from build123d import *

# Parameters (mm, degrees)
BOSS_EXTRUDE1_DEPTH                            = 6.35
CSK_FOR_4_FLAT_HEAD_MACHINE_SCREW1_D           = 3.2639
CSK_FOR_4_FLAT_HEAD_MACHINE_SCREW1_CSINK_D     = 5.715
CSK_FOR_4_FLAT_HEAD_MACHINE_SCREW1_CSINK_ANGLE = 82
CSK_FOR_4_FLAT_HEAD_MACHINE_SCREW2_D           = 3.2639
CSK_FOR_4_FLAT_HEAD_MACHINE_SCREW2_CSINK_D     = 5.715
CSK_FOR_4_FLAT_HEAD_MACHINE_SCREW2_CSINK_ANGLE = 82
CHAMFER1_SIZE                                  = 10.558581723
CHAMFER1_SIZE_2                                = 6.096
CUT_EXTRUDE1_REACH                             = 697.184
SKETCH8_W                                      = 25.4
SKETCH8_H                                      = 49.00517421
CSK_FOR_4_FLAT_HEAD_MACHINE_SCREW3_D           = 3.2639
CSK_FOR_4_FLAT_HEAD_MACHINE_SCREW3_CSINK_D     = 5.715
CSK_FOR_4_FLAT_HEAD_MACHINE_SCREW3_CSINK_ANGLE = 82


with BuildPart() as part:
    # Sketch1 → Boss-Extrude1 (new body)
    with BuildSketch(Plane(origin=(0, 0, 0), x_dir=(0, 0, -1), z_dir=(1, 0, 0))):
        with BuildLine():
            Line((-123.515928009, -106.162611625), (-0.699091996, 106.562388375))
            ThreePointArc((-0.699091996, 106.562388375), (110.865451078, 218.126931449), (263.265451078, 258.962388375))
            Line((263.265451078, 258.962388375), (646.089089029, 258.962388375))
            Line((646.089089029, 258.962388375), (646.089089029, -106.162611625))
            Line((646.089089029, -106.162611625), (-123.515928009, -106.162611625))
        make_face()
    extrude(amount=BOSS_EXTRUDE1_DEPTH)

    # CSK for #4 Flat Head Machine Screw1 (through all)
    with Locations(Plane(origin=(6.35, 0, 0), x_dir=(0, 0, -1), z_dir=(1, 0, 0))):
        with Locations((633.389089029, 29.727388375)):
            CounterSinkHole(CSK_FOR_4_FLAT_HEAD_MACHINE_SCREW1_D / 2, CSK_FOR_4_FLAT_HEAD_MACHINE_SCREW1_CSINK_D / 2, counter_sink_angle=CSK_FOR_4_FLAT_HEAD_MACHINE_SCREW1_CSINK_ANGLE)

    # CSK for #4 Flat Head Machine Screw2 (through all)
    with Locations(Plane(origin=(6.35, 207.527388375, -315.889089029), x_dir=(0, 0, 1), z_dir=(1, 0, 0))):
        with Locations((0, 0), (-317.5, 25.4)):
            CounterSinkHole(CSK_FOR_4_FLAT_HEAD_MACHINE_SCREW2_D / 2, CSK_FOR_4_FLAT_HEAD_MACHINE_SCREW2_CSINK_D / 2, counter_sink_angle=CSK_FOR_4_FLAT_HEAD_MACHINE_SCREW2_CSINK_ANGLE)

    # Chamfer1
    # the kernel refuses this chamfer: 10.558581723, 6.096 mm, written as the material it takes off along each edge
    with BuildSketch(Plane(origin=(0, -129.818923765, 137.173906191), x_dir=(0.9998132206222078, 0.009663382806350982, 0.016737469993587533), z_dir=(0, 0.8660254037844402, -0.49999999999999756))) as chamfer1_piece_1:
        Polygon((CHAMFER1_SIZE * 0.999813220617, CHAMFER1_SIZE * 0.0193267656126), (-CHAMFER1_SIZE_2 * 0.0193267656127, CHAMFER1_SIZE_2 * 0.999813220622), (0, 0), align=None)
    extrude(amount=272.949628391, mode=Mode.SUBTRACT)
    with BuildSketch(Plane(origin=(0, -45.837611625, -263.265451078), x_dir=(0, 0.5000000000000027, 0.8660254037844372), z_dir=(0, -0.8660254037844372, 0.5000000000000027))) as chamfer1_piece_2:
        Polygon((304.8 - CHAMFER1_SIZE_2, 0), (304.8, -CHAMFER1_SIZE), (304.8, 0), align=None)
    revolve(axis=Axis((0, -45.837611625, -263.265451078), (-1, 0, 0)), revolution_arc=60, mode=Mode.SUBTRACT)
    with BuildSketch(Plane(origin=(0, 258.962388375, -263.265451078), x_dir=(0.9998132206222078, 0.01932676561270281, 0), z_dir=(0, 0, -1))) as chamfer1_piece_3:
        Polygon((CHAMFER1_SIZE * 0.999813220617, CHAMFER1_SIZE * 0.0193267656126), (-CHAMFER1_SIZE_2 * 0.0193267656127, CHAMFER1_SIZE_2 * 0.999813220622), (0, 0), align=None)
    extrude(amount=410.139594316, mode=Mode.SUBTRACT)

    # Sketch8 → Cut-Extrude1 (cut, up to next)
    with BuildSketch(Plane(origin=(6.35, 0, 0), x_dir=(0, 0, -1), z_dir=(1, 0, 0)), mode=Mode.PRIVATE) as cut_extrude1_sk1:
        with Locations((623.864089029, 232.02997548)):
            Rectangle(SKETCH8_W, SKETCH8_H)
    cut_extrude1_tool1 = extrude(cut_extrude1_sk1.sketch, amount=-CUT_EXTRUDE1_REACH, mode=Mode.PRIVATE) & part.part
    add(cut_extrude1_tool1.solids().sort_by_distance((6.35, 232.029975, -623.864089))[0], mode=Mode.SUBTRACT)

    # CSK for #4 Flat Head Machine Screw3 (through all)
    with Locations(Plane(origin=(6.35, -80.762611625, -569.889089029), x_dir=(0, 0, 1), z_dir=(1, 0, 0))):
        with Locations((0, 0), (228.6, 0)):
            CounterSinkHole(CSK_FOR_4_FLAT_HEAD_MACHINE_SCREW3_D / 2, CSK_FOR_4_FLAT_HEAD_MACHINE_SCREW3_CSINK_D / 2, counter_sink_angle=CSK_FOR_4_FLAT_HEAD_MACHINE_SCREW3_CSINK_ANGLE)


solid = part.part
CAD build for the part. Positions are in the model's coordinates, mm. Round coordinates to 2 decimals unless told otherwise and drop trailing zeros. Order: outer loops, then holes, each group sorted by start corner. A loop starts at its lowest first (then second) coordinate and runs counter-clockwise, first axis right, second up. Notation, with made-up numbers: (49.5, 39.25) - (82.5, 39.25) arc R37 ccw to (82.5, 75.25) - close; hole circle Ø11 at (82, 33.25). An arc over 180 degrees is marked (long way). Return JSON: item names as keys, results as strings.
(1) Pin check, flat tips, straight feed: pin 1 Ø3 at (x, z) = (3, -624) entering from +Y; pin 2 Ø4 at (y, z) = (29.73, -633.39) entering from +X. Stop position of each tip, or through.
Answer key:
{"pin 1": "stops at y = 207.53", "pin 2": "stops at x = 5.37"}
(2) Cut at A-A (x = 2.5). Give the cut face in (y, z).
Answer key:
{"outline": "(-106.16, -646.09) - (254.31, -646.09) - (254.31, -636.56) - (207.53, -636.56) - (207.53, -611.16) - (254.31, -611.16) - (254.31, -263.27) arc R300.15 ccw to (104.24, -3.33) - (-106.16, 118.14) - close; hole circle Ø3.26 at (-80.76, -569.89); hole circle Ø3.26 at (-80.76, -341.29); hole circle Ø3.26 at (29.73, -633.39); hole circle Ø3.26 at (182.13, -633.39); hole circle Ø3.26 at (207.53, -315.89)"}
(3) Wall check: probe 1 along Z at (x, y) = (4, 212.5); probe 2 along Y at (x, z) = (0.5, -320.5); probe 3 along Z at (x, y) = (6.25, 134). Give the ranges that are in metal, low to high. Write a range as from..to.
Answer key:
{"probe 1": "z = -646.09..-636.56, -611.16..-108.76", "probe 2": "y = -106.16..253.16", "probe 3": "z = -646.09..-20.26"}
(4) Cut at B-B (y = 4.5). Give the cut face in (x, z), then the cut area to 3 significant figures.
Answer key:
{"outline": "(0, -646.09) - (6.35, -646.09) - (6.35, 56.82) - (0, 52.59) - close", "area": "4,450 mm^2"}
